Here's how the part is built. I have some questions about the finished solid (model axes, mm). Face numbers are marked on the shaded views. A direction names the side the tool comes from. Coordinates: 2 decimals unless noted, no trailing zeros. Put each result on its own line as item: value. Start each with the question number.
Item 1: On a 3-axis mill with a long thin cutter (end or side, diameter ignored), from which of +Z, -Z, +X, -X, +Y, -Y can I reach the whole of each face in a straight line? I mean the marked faces 1, 2 and 3. Say none if no direction works.
Item 2: If we mould it in two halves opening along Z, with no side actions, what happens to the marked faces 4, 5 and 6? For each: released by +Z, released by -Z, zero draft, split by the parting line, or undercut.
Item 3: I want a section at A-A, the plane y = -7.5. State how many separate pieces and enclosed holes the cut face has, then the cut area to 3 significant figures.
Item 4: I need wall thicknesses on line 1 (X direction, y = -6, z = 2.5); line 2 (Y direction, x = 13.5, z = 6); line 3 (Z direction, x = 3.5, y = -4). Which ranges of each line are inside material? Lowest first, please. Write a range as [from, to].
Item 5: For pin 1 (1 mm diameter, centred on y = -10.5, z = 8, fed in from +X); pin 2 (1.4 mm diameter, centred on y = -4, z = 6, fed in from +X); pin 3 (0.6 mm diameter, centred on x = -3, z = 6.5, fed in from +Y); pin 4 (5.5 mm diameter, centred on x = 9.5, y = 3.5, fed in from +Z), each with a flat end and sliding along its axis, tell me the tip position at first contact or that it passes through.
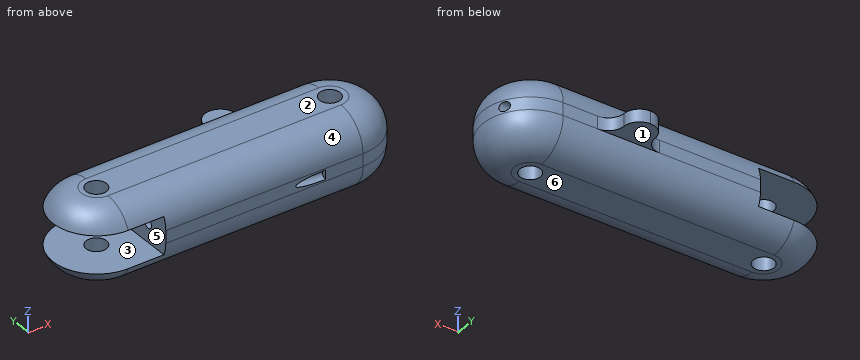
from build123d import *

# Parameters (mm, degrees)
BOSS_EXTRUDE1_DEPTH = 12
FILLET1_R           = 5
SKETCH5_W           = 13.25
SKETCH5_H           = 6
CUT_EXTRUDE3_DEPTH  = 39.184584586
SKETCH6_W           = 5
SKETCH6_H           = 2
BOSS_EXTRUDE2_DEPTH = 5
FILLET2_R           = 2.5
FILLET3_R           = 2.5
SKETCH3_R           = 1.65
CUT_EXTRUDE4_DEPTH  = 33.5278727
SKETCH8_R           = 0.75
CUT_EXTRUDE7_DEPTH  = 56.512113127
SKETCH9_R           = 0.75
CUT_EXTRUDE9_DEPTH  = 26.058827679


with BuildPart() as part:
    # Sketch2 → Boss-Extrude1 (new body)
    with BuildSketch(Plane.XY):
        with BuildLine():
            Line((-18.75, 0), (18.75, 0))
            ThreePointArc((18.75, 0), (26.25, -7.5), (18.75, -15))
            Line((18.75, -15), (-18.75, -15))
            ThreePointArc((-18.75, -15), (-26.25, -7.5), (-18.75, 0))
        make_face()
    extrude(amount=BOSS_EXTRUDE1_DEPTH)

    # Fillet1
    fillet1_edges = [part.edges().sort_by_distance(p)[0] for p in [
        (-26.25, -7.5, 12),
        (0, -15, 12),
        (26.25, -7.5, 12),
        (0, -15, 0),
        (-26.25, -7.5, 0),
        (0, 0, 0),
        (26.25, -7.5, 0),
        (0, 0, 12),
    ]]
    fillet(fillet1_edges, radius=FILLET1_R)

    # Sketch5 → Cut-Extrude3 (cut, through all)
    with BuildSketch(Plane(origin=(0, -25, 0), x_dir=(-1, 0, 0), z_dir=(0, -1, 0))):
        with Locations((19.625, -6)):
            Rectangle(SKETCH5_W, SKETCH5_H)
    extrude(amount=-CUT_EXTRUDE3_DEPTH, mode=Mode.SUBTRACT)

    # Sketch6 → Boss-Extrude2 (add)
    with BuildSketch(Plane(origin=(0, 0, 0), x_dir=(1, 0, 0), z_dir=(0, 1, 0))):
        with Locations((8.25, -6)):
            Rectangle(SKETCH6_W, SKETCH6_H)
    extrude(amount=BOSS_EXTRUDE2_DEPTH)

    # Fillet2
    fillet2_edges = [part.edges().sort_by_distance(p)[0] for p in [
        (10.75, 5, 6),
        (5.75, 5, 6),
    ]]
    fillet(fillet2_edges, radius=FILLET2_R - 0.0001)  # a hair under: the kernel refuses the full size

    # Fillet3
    fillet3_edges = [part.edges().sort_by_distance(p)[0] for p in [
        (5.75, 0, 6),
        (10.75, 0, 6),
    ]]
    fillet(fillet3_edges, radius=FILLET3_R)

    # Sketch3 → Cut-Extrude4 (cut, through all)
    with BuildSketch(Plane.XY.offset(12)):
        with Locations((-18.853477977, -7.5)):
            Circle(SKETCH3_R)
        with Locations((18.75, -7.5)):
            Circle(SKETCH3_R)
    extrude(amount=-CUT_EXTRUDE4_DEPTH, mode=Mode.SUBTRACT)

    # Sketch8 → Cut-Extrude7 (cut, through all)
    with BuildSketch(Plane(origin=(26.25, 0, 0), x_dir=(0, 0, -1), z_dir=(1, 0, 0))):
        with Locations((-6, -4)):
            Circle(SKETCH8_R)
    extrude(amount=-CUT_EXTRUDE7_DEPTH, mode=Mode.SUBTRACT)

    # Sketch9 → Cut-Extrude9 (cut, along a direction that is not the sketch's normal)
    with BuildSketch(Plane.ZY.offset(13)):
        with Locations((6, -11)):
            Circle(SKETCH9_R)
    extrude(amount=-CUT_EXTRUDE9_DEPTH, dir=(-0.988148826849317, 0.15349884688921422, 0), mode=Mode.SUBTRACT)


solid = part.part
Calculated:
1. face 1: -Z, +X, -X, +Y
1. face 2: +Z, +X, -X, +Y, -Y
1. face 3: -X, +Y, -Y
2. face 4: released by +Z
2. face 5: undercut
2. face 6: released by -Z
3. separate pieces: 4
3. enclosed holes: 0
3. area: 470 mm2
4. line 1: x = [-25.41, -19.54], [-18.17, 18.06], [19.44, 25.41]
4. line 2: y = [-15, -4.75], [-3.25, 0]
4. line 3: z = [0.1, 5.25], [6.75, 11.9]
5. pin 1: stops at x = 25.74
5. pin 2: passes through
5. pin 3: stops at y = 0
5. pin 4: stops at z = 7
